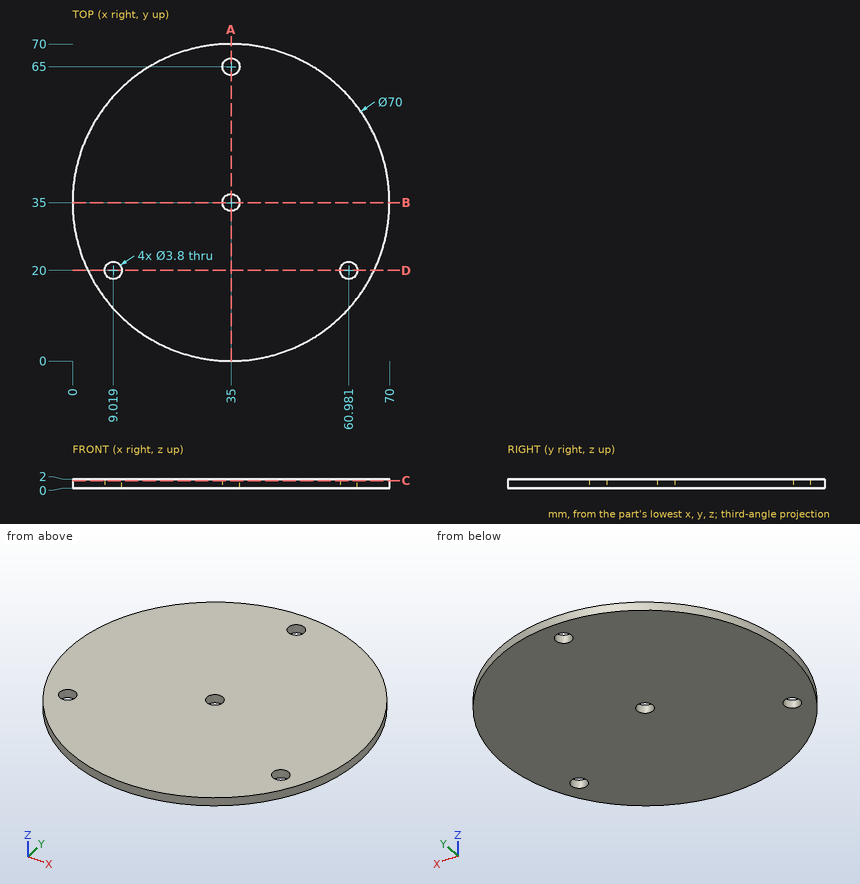
Source: three-view drawing plus pictorial views. Frame: mm from the lowest corner of the part. Round coordinates to 2 decimals unless told otherwise and drop trailing zeros. Loops run counter-clockwise (first coordinate to the right, second up) from the corner with the lowest first, then second, coordinate; pieces in that order, holes last. Notation, with made-up numbers: (51.25, 5.5) - (74.25, 5.5) arc R34 cw to (74.25, 41.5) - close; hole circle Ø3 at (-35.5, 80.25). An arc over 180 degrees is marked (long way). Write each question's results on one line, items separated by ' | '. Start each with the question number.
1) Cut plane B-B on y = 35. Return loops of the section in (x, z), then the cut area to 3 significant figures.
2) Line query: probe 1 along Y at (x, z) = (35, 0.9); probe 2 along X at (y, z) = (20, 1); probe 3 along Y at (x, z) = (62, 1.05) (1 decimal). Output: solid intervals per line, ascending. Write a range as [from, to].
3) First-contact query: P1, Ø1, axis at y = 52, z = 1, coming from the +X side; P2, Ø3.5, axis at x = 35, y = 35, coming from the -Z side. Flat tips, straight axial feed; report the tip coordinate or a pass-through.
4) Cut plane D-D on y = 20. Return loops of the section in (x, z), then the cut area to 3 significant figures.
5) Cut plane C-C on z = 1.65. Return loops of the section in (x, y), then the cut area to 3 significant figures.
6) Cut plane A-A on x = 35. Return loops of the section in (y, z).
Verdict:
1) outline: (0, 0) - (33.1, 0) - (33.1, 2) - (0, 2) - close; (36.9, 0) - (70, 0) - (70, 2) - (36.9, 2) - close | area: 132 mm2
2) probe 1: y = [0, 33.1], [36.9, 63.1], [66.9, 70] | probe 2: x = [3.38, 7.12], [10.92, 59.08], [62.88, 66.62] | probe 3: y = [12.7, 18.4], [21.6, 57.3]
3) P1: stops at x = 65.87 | P2: passes through
4) outline: (3.38, 0) - (7.12, 0) - (7.12, 2) - (3.38, 2) - close; (10.92, 0) - (59.08, 0) - (59.08, 2) - (10.92, 2) - close; (62.88, 0) - (66.62, 0) - (66.62, 2) - (62.88, 2) - close | area: 111 mm2
5) outline: circle Ø70 at (35, 35); hole circle Ø3.8 at (9.02, 20); hole circle Ø3.8 at (35, 35); hole circle Ø3.8 at (35, 65); hole circle Ø3.8 at (60.98, 20) | area: 3,800 mm2
6) outline: (0, 0) - (33.1, 0) - (33.1, 2) - (0, 2) - close; (36.9, 0) - (63.1, 0) - (63.1, 2) - (36.9, 2) - close; (66.9, 0) - (70, 0) - (70, 2) - (66.9, 2) - close
